Source: three-view drawing plus pictorial views. Frame: mm from the lowest corner of the part. A direction names the side the tool comes from. Give positions to 0.01 mm unless a question says otherwise; leave off trailing zeros. Write each loop counter-clockwise with the first axis right and the second up, starting at its lowest first coordinate (ties: lowest second). Pieces come first, ordered by that corner, then holes.
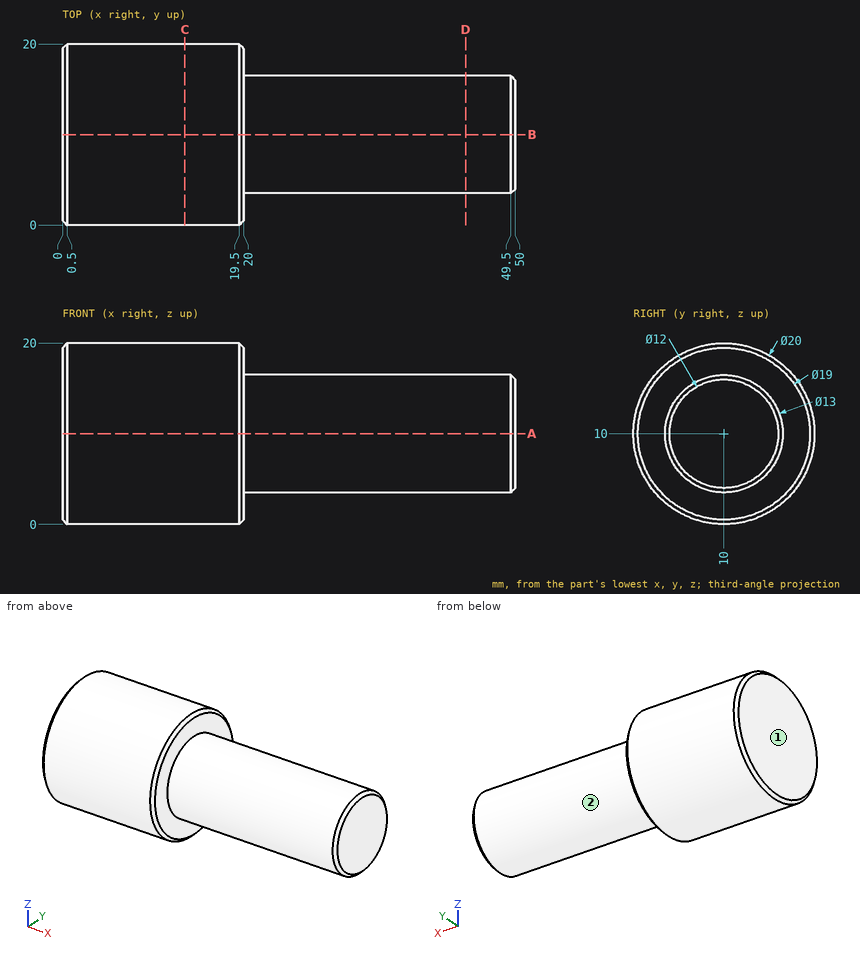
Q1. Ray query, line 1 along X through (y, z) = (14.5, 2); line 2 along Z through (x, y) = (31, 10.25); line 3 along Y through (x, z) = (17, 7). Return the intervals inside material, ascending.
Filled sheet:
line 1: x = 0 to 20
line 2: z = 3.5 to 16.5
line 3: y = 0.46 to 19.54
Q2. Section A-A on z = 10. Output: boundary loops of the cut face in (x, y), plus the area to 3 significant figures.
Filled sheet:
outline: (0, 0.5) - (0.5, 0) - (19.5, 0) - (20, 0.5) - (20, 3.5) - (49.5, 3.5) - (50, 4) - (50, 16) - (49.5, 16.5) - (20, 16.5) - (20, 19.5) - (19.5, 20) - (0.5, 20) - (0, 19.5) - close
area: 789 mm2
Q3. Section D-D on x = 44.5. Output: boundary loops of the cut face in (y, z), plus the area to 3 significant figures.
Filled sheet:
outline: circle Ø13 at (10, 10)
area: 133 mm2
Q4. Access query for the marked faces 1 and 2. Directions: +Z, -Z, +X, -X, +Y, -Y. A direction counts if a zero-diameter tool reaches every point of the face in a straight line with its end or side. Return the directions, or none.
Filled sheet:
face 1: +Z, -Z, -X, +Y, -Y
face 2: +X
Q5. Section C-C on x = 13.5. Output: boundary loops of the cut face in (y, z), plus the area to 3 significant figures.
Filled sheet:
outline: circle Ø20 at (10, 10)
area: 314 mm2
Q6. Pin query (flat end, axial travel): P1, Ø4, axis at x = 13.5, y = 17, coming from the +Z side; P2, Ø1.5, axis at x = 29.5, z = 13.5, coming from the +Y side; P3, Ø5, axis at x = 5, y = 17, coming from the +Z side. Return the tip coordinate at first contact, or that it passes through.
Filled sheet:
P1: stops at z = 18.66
P2: stops at y = 15.89
P3: stops at z = 18.93
